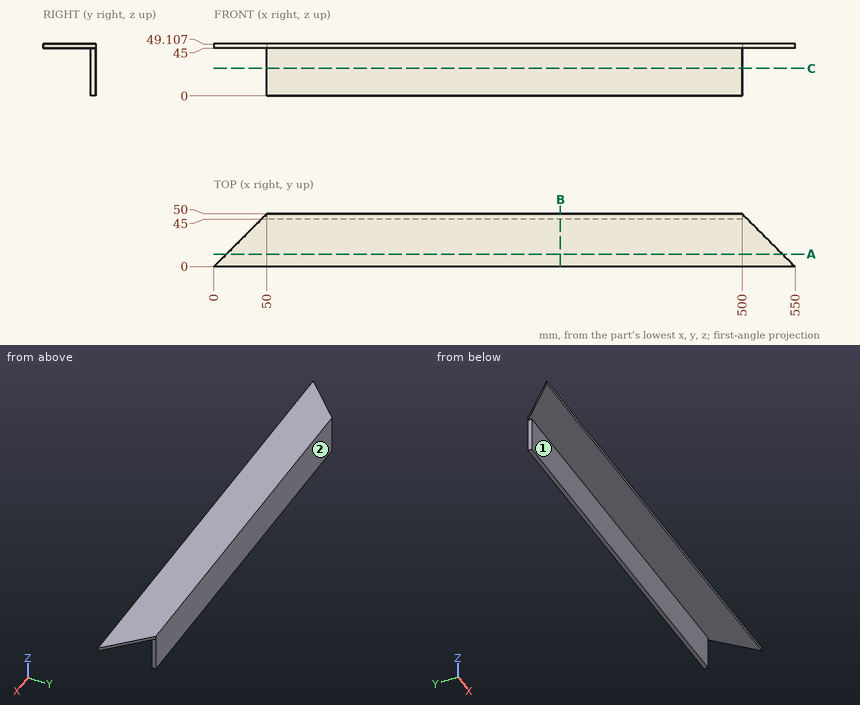
Could you check a few things on this drawing? It's one solid part, dimensions in mm from its lowest x, y, z. A direction names the side the tool comes from. Coordinates: 2 decimals unless noted, no trailing zeros. Order: outer loops, then holes, each group sorted by start corner. A loop starts at its lowest first (then second) coordinate and runs counter-clockwise, first axis right, second up. Notation, with made-up numbers: M -35,48.25 L 24,48.25 A27 cw 24,81.25 Z; hole C 58,-12 d3. An arc over 180 degrees is marked long. Answer as CSV lines item,"result".
(1) I'm going to push flat-ended pins straight in: pin 1 (1.5 mm diameter, centred on y = 47, z = 33.5, fed in from -X); pin 2 (8 mm diameter, centred on y = 40.5, z = 36, fed in from +X); pin 3 (10 mm diameter, centred on x = 164, y = 25, fed in from -Z); pin 4 (1.5 mm diameter, centred on y = 47, z = 27.5, fed in from +X). Where does each tip first touch, or does it pass through?
Geometry check:
pin 1,"x = 50"
pin 2,"through"
pin 3,"z = 45"
pin 4,"x = 500"
(2) Suppose I cut it at B-B on x = 328. Please give me the cut outline in (y, z).
Geometry check:
outline,"M 0,45 L 45,45 L 45,0 L 50,0 L 50,49.11 L 0,49.11 Z"
(3) Please list where these lines run through material, in increasing order: L1, parallel to Y at x = 95, z = 36; L2, parallel to Z at x = 324.5, y = 15.
Geometry check:
L1,"45 to 50"
L2,"45 to 49.11"
(4) Suppose I cut it at A-A on y = 12. Please give me the cut outline in (x, z).
Geometry check:
outline,"M 12,45 L 538,45 L 538,49.11 L 12,49.11 Z"
(5) On a 3-axis mill with a long thin cutter (end or side, diameter ignored), from which of +Z, -Z, +X, -X, +Y, -Y can I reach the whole of each face in a straight line? I mean the marked faces 1 and 2. Say none if no direction works.
Geometry check:
face 1,"-Z, +X, -X, -Y"
face 2,"+Z, -Z, +X, -X, +Y"
(6) Suppose I cut it at C-C on z = 26. Please give me the cut outline in (x, y), plus the area to 3 significant figures.
Geometry check:
outline,"M 50,45 L 500,45 L 500,50 L 50,50 Z"
area,"2,250 mm^2"
